from build123d import *


with BuildPart() as part:
    # Sketch2 → Revolve1 (revolve)
    with BuildSketch(Plane.XY, mode=Mode.PRIVATE) as revolve1_sk:
        with BuildLine():
            Line((0.45, 0.423325242), (0.45, 15.423325242))
            Line((0.45, 15.423325242), (15.45, 15.423325242))
            Line((15.45, 15.423325242), (15.45, 0.423325242))
            Line((15.45, 0.423325242), (2.35, 0.423325242))
            Line((2.35, 0.423325242), (2.35, 1.206680612))
            Line((2.35, 1.206680612), (2.32901869, 3.903053406))
            Line((2.32901869, 3.903053406), (2.32901869, 8.430876594))
            add(Edge.make_bspline(
                [(4.196605338, 10.969687667), (3.922502386, 11.441848149), (2.509035232, 10.990794392), (2.220509348, 9.330364972), (2.32901869, 8.430876594)],
                knots=[0, 0, 0, 0, 0.262564072, 1, 1, 1, 1], degree=3))
            Line((4.196605338, 10.969687667), (4.778131503, 7.236007047))
            ThreePointArc((4.778131503, 7.236007047), (6.500210622, 4.147064861), (9.817375473, 2.920876594))
            Line((9.817375473, 2.920876594), (11.307027571, 2.920876594))
            ThreePointArc((11.307027571, 2.920876594), (11.826873824, 2.945454106), (12.342082499, 3.018967384))
            Line((12.342082499, 3.018967384), (13.489606212, 3.238437081))
            ThreePointArc((13.489606212, 3.238437081), (13.619163994, 3.281851358), (13.732545298, 3.358105526))
            Line((13.732545298, 3.358105526), (13.788115607, 3.407479744))
            ThreePointArc((13.788115607, 3.407479744), (14.308903284, 4.116856602), (14.493292649, 4.977342449))
            Line((14.493292649, 4.977342449), (14.493292649, 9.039992195))
            Line((14.493292649, 9.039992195), (7.825729831, 9.039992195))
            add(Edge.make_bspline(
                [(0.9, 11.277873829), (1.154261749, 13.796749585), (3.412741165, 15.062987228), (6.394883753, 13.664649552), (6.379029002, 12.127449794), (6.776722254, 10.540030851), (6.74201353, 9.221561674), (7.825729831, 9.039992195)],
                knots=[0, 0, 0, 0, 0.440870588, 0.577759513, 0.724851521, 0.783369034, 1, 1, 1, 1], degree=3))
            Line((0.9, 11.277873829), (0.9, 0.423325242))
            Line((0.9, 0.423325242), (0.45, 0.423325242))
        make_face()
    revolve(revolve1_sk.sketch.rotate(Axis((0, 28.78036469, 0), (0, -1, 0)), 90), axis=Axis((0, 28.78036469, 0), (0, -1, 0)))


solid = part.part
Could you check a few things on this model? Use its own coordinates, in mm. A direction names the side the tool comes from. Give positions to 0.01 mm unless a question says otherwise; leave off trailing zeros. Order: outer loops, then holes, each group sorted by start corner. A loop starts at its lowest first (then second) coordinate and runs counter-clockwise, first axis right, second up. Notation, with made-up numbers: (8, -16.5) -> (25, -16.5) arc R38 cw to (25, 22.5) -> close; hole circle Ø10 at (-1.5, 12.25). An arc over 180 degrees is marked (long way). Answer in a Markdown table with one row per item. Add a question column.
Item 1: Imagine slicing it at B-B (y = 2.25). List the corners of the cut face in (x, z) for me, and give its area (3 significant figures).
Item 2: Please list where these lines run through material, in increasing order: probe 1 along X at (y, z) = (0.8, 0); probe 2 along X at (y, z) = (9.5, -2.5); probe 3 along X at (y, z) = (6.25, -4).
Item 3: Imagine slicing it at A-A (y = 5.5). List the corners of the cut face in (x, z) for me.
Item 4: We'd pull the mould along Z, two halves only. Please class faces 1 (the cylindrical face through (2.274, 6.199, -0.505)), 2 (the cylindrical face through (13.707, 7.818, 7.129)), 3 (the flat face through (0, 15.423, -3)): pulls with the +Z half, pulls with the -Z half, needs draft (parallel to the pull), parting line crosses it, or undercut.
Item 5: I'm going to push flat-ended pins straight in: P1, Ø6, axis at x = -8.5, y = 6, coming from the -Z side; P2, Ø5, axis at x = 4.5, y = 13.5, coming from the +Z side; P3, Ø8, axis at y = 12.5, z = -11.5, coming from the -X side. Where does each tip first touch, or does it pass through?
Item 6: Imagine slicing it at C-C (y = 13.25). Count the separate pieces of the cut face and the enclosed holes in it, and give its area (3 significant figures).
Item 7: For faces 4 (the flat face through (-10, 2.921, 0)), 5 (the cylindrical face through (-0.135, 8.028, 0.429)), 6 (the cylindrical face through (2.294, 0.82, -0.509)), which set-ups out of +Z, -Z, +X, -X, +Y, -Y let a thin tool reach every point of the face, with its end or its side?
Result:
| question | item | result |
|---|---|---|
| 1 | outline | circle Ø30.9 at (0, 0); circle Ø1.8 at (0, 0); hole circle Ø4.68 at (0, 0); hole circle Ø0.9 at (0, 0) |
| 1 | area | 735 mm2 |
| 2 | probe 1 | -15.45 to -2.35, -0.9 to -0.45, 0.45 to 0.9, 2.35 to 15.45 |
| 2 | probe 2 | -15.25 to -6.58, -3.65 to 3.65, 6.58 to 15.25 |
| 2 | probe 3 | -14.92 to -13.93, -3.06 to 3.06, 13.93 to 14.92 |
| 3 | outline | circle Ø30.9 at (0, 0); circle Ø10.77 at (0, 0); circle Ø1.8 at (0, 0); hole circle Ø28.99 at (0, 0); hole circle Ø4.66 at (0, 0); hole circle Ø0.9 at (0, 0) |
| 4 | face 1 | undercut |
| 4 | face 2 | parting line crosses it |
| 4 | face 3 | needs draft |
| 5 | P1 | z = -14.44 |
| 5 | P2 | z = 15.32 |
| 5 | P3 | x = -13.51 |
| 6 | separate pieces | 2 |
| 6 | enclosed holes | 2 |
| 6 | area | 636 mm2 |
| 7 | face 4 | none |
| 7 | face 5 | +Y, -Y |
| 7 | face 6 | -Y |
